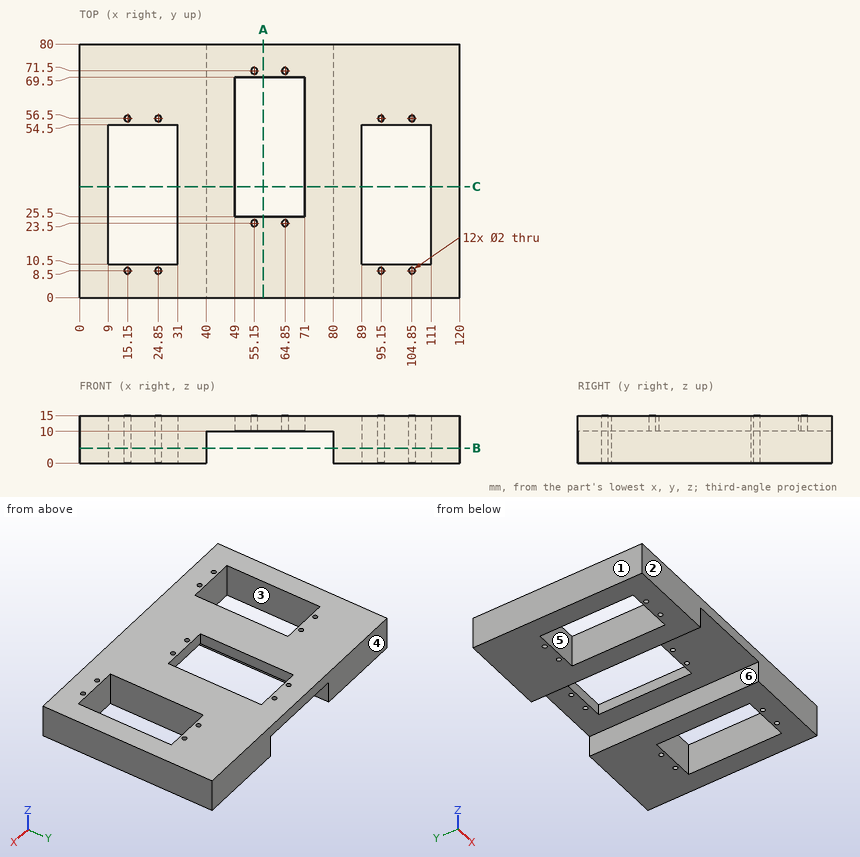
Study the drawing (mm; zero at the part's minimum x, y, z) and answer. A direction names the side the tool comes from. Coordinates: 2 decimals unless noted, no trailing zeros. Order: outer loops, then holes, each group sorted by start corner. A loop starts at its lowest first (then second) coordinate and runs counter-clockwise, first axis right, second up. Notation, with made-up numbers: (-7.75, -38.75) -> (40.25, -38.75) arc R16 ccw to (40.25, -16.75) -> close; hole circle Ø9 at (25.5, 17.5). An arc over 180 degrees is marked (long way). Answer in a Markdown table with one row per item. Add a question column.
Item 1: Find section A-A (x = 58). Write down the section's boundary in (y, z).
Item 2: Which of the six approach directions +Z, -Z, +X, -X, +Y, -Y give full straight-line access (tool end or side, diameter ignored) to the marked faces 4, 5 and 6?
Item 3: Each of these flat-tipped pins is pushed along its axis until it touches: P1, Ø3, axis at x = 24.85, y = 56.5, coming from the +Z side; P2, Ø12, axis at x = 62.5, y = 50, coming from the -Z side; P3, Ø3, axis at x = 55.15, y = 23.5, coming from the -Z side. Where does it stop, or does it pass through?
Item 4: Find section C-C (y = 35). Write down the section's boundary in (x, z), then the cut area to 3 significant figures.
Item 5: Find section B-B (z = 4.75). State how many separate pieces and enclosed holes the cut face has, then the cut area to 3 significant figures.
Item 6: Determine the mould class of the marked faces 1, 2 and 3 for opening direction Y: +Y half, -Y half, draft (parallel to the pull), parting line (faces both ways), or undercut.
Item 7: Find the intervals of material crossed by L1, parallel to X at y = 18, z = 8.5; L2, parallel to Y at x = 55.15, z = 12.1; L3, parallel to Y at x = 104.85, z = 8.25, in increasing order. Write a range as from..to.
Result set:
| question | item | result |
|---|---|---|
| 1 | outline | (0, 10) -> (25.5, 10) -> (25.5, 15) -> (0, 15) -> close; (69.5, 10) -> (80, 10) -> (80, 15) -> (69.5, 15) -> close |
| 2 | face 4 | +Z, -Z, +X, -X, +Y |
| 2 | face 5 | +Z, -Z |
| 2 | face 6 | -Z, +Y, -Y |
| 3 | P1 | stops at z = 15 |
| 3 | P2 | passes through |
| 3 | P3 | stops at z = 10 |
| 4 | outline | (0, 0) -> (9, 0) -> (9, 15) -> (0, 15) -> close; (31, 0) -> (40, 0) -> (40, 10) -> (49, 10) -> (49, 15) -> (31, 15) -> close; (71, 10) -> (80, 10) -> (80, 0) -> (89, 0) -> (89, 15) -> (71, 15) -> close; (111, 0) -> (120, 0) -> (120, 15) -> (111, 15) -> close |
| 4 | area | 630 mm² |
| 5 | separate pieces | 2 |
| 5 | enclosed holes | 10 |
| 5 | area | 4,440 mm² |
| 6 | face 1 | draft |
| 6 | face 2 | -Y half |
| 6 | face 3 | undercut |
| 7 | L1 | x = 0..9, 31..40, 80..89, 111..120 |
| 7 | L2 | y = 0..22.5, 24.5..25.5, 69.5..70.5, 72.5..80 |
| 7 | L3 | y = 0..7.5, 9.5..10.5, 54.5..55.5, 57.5..80 |
